Geometry check sheet. Reference: the model listing, model coordinates, mm. Give positions to 0.01 mm unless a question says otherwise; leave off trailing zeros. Loops run counter-clockwise (first coordinate to the right, second up) from the corner with the lowest first, then second, coordinate; pieces in that order, holes last. Notation, with made-up numbers: (-19, 36.25) -> (-9, 36.25) arc R24 cw to (-9, 64.25) -> close; hole circle Ø8 at (11.25, 69.5). An arc over 180 degrees is marked (long way). Answer as a JSON object with one key per item and string values.
from build123d import *

# Parameters (mm, degrees)
BOSS_EXTRUDE1_DEPTH = 1.15
CUT_EXTRUDE1_REACH  = 3.15
SKETCH2_R           = 1.55
SKETCH3_W           = 5.45
SKETCH3_H           = 4.15
BOSS_EXTRUDE2_DEPTH = 2.3
SKETCH4_W           = 9.718661505
SKETCH4_H           = 9.252165754
SKETCH4_W_2         = 4.664957522
SKETCH4_H_2         = 2.876723805
SKETCH4_W_3         = 4.081837833
SKETCH4_H_3         = 2.798974514
SKETCH4_W_4         = 4.159587124
SKETCH4_H_4         = 1.593860487
SKETCH4_W_5         = 2.64347593
SKETCH4_H_5         = 0.971866151
BOSS_EXTRUDE3_DEPTH = 1


with BuildPart() as part:
    # Sketch1 → Boss-Extrude1 (new body)
    with BuildSketch(Plane(origin=(0, 0, 0), x_dir=(1, 0, 0), z_dir=(0, 1, 0))):
        with BuildLine():
            Line((-19.425, 20.3), (19.425, 20.3))
            ThreePointArc((19.425, 20.3), (20.839213562, 19.714213562), (21.425, 18.3))
            Line((21.425, 18.3), (21.425, -18.3))
            ThreePointArc((21.425, -18.3), (20.839213562, -19.714213562), (19.425, -20.3))
            Line((19.425, -20.3), (-19.425, -20.3))
            ThreePointArc((-19.425, -20.3), (-20.839213562, -19.714213562), (-21.425, -18.3))
            Line((-21.425, -18.3), (-21.425, 18.3))
            ThreePointArc((-21.425, 18.3), (-20.839213562, 19.714213562), (-19.425, 20.3))
        make_face()
    extrude(amount=BOSS_EXTRUDE1_DEPTH)

    # Sketch2 → Cut-Extrude1 (cut, up to next)
    with BuildSketch(Plane(origin=(0, 1.15, 0), x_dir=(1, 0, 0), z_dir=(0, 1, 0)), mode=Mode.PRIVATE) as cut_extrude1_sk1:
        with Locations((-13.925, 12.95)):
            Circle(SKETCH2_R)
    cut_extrude1_tool1 = extrude(cut_extrude1_sk1.sketch, amount=-CUT_EXTRUDE1_REACH, mode=Mode.PRIVATE) & part.part
    add(cut_extrude1_tool1.solids().sort_by_distance((-13.925, 1.15, -12.95))[0], mode=Mode.SUBTRACT)
    # Sketch2 → Cut-Extrude1 (cut, up to next)
    with BuildSketch(Plane(origin=(0, 1.15, 0), x_dir=(1, 0, 0), z_dir=(0, 1, 0)), mode=Mode.PRIVATE) as cut_extrude1_sk2:
        with Locations((13.925, -12.95)):
            Circle(SKETCH2_R)
    cut_extrude1_tool2 = extrude(cut_extrude1_sk2.sketch, amount=-CUT_EXTRUDE1_REACH, mode=Mode.PRIVATE) & part.part
    add(cut_extrude1_tool2.solids().sort_by_distance((13.925, 1.15, 12.95))[0], mode=Mode.SUBTRACT)

    # Sketch3 → Boss-Extrude2 (add)
    with BuildSketch(Plane(origin=(0, 1.15, 0), x_dir=(1, 0, 0), z_dir=(0, 1, 0))):
        with Locations((-9.84, -9.405)):
            Rectangle(SKETCH3_W, SKETCH3_H)
    extrude(amount=BOSS_EXTRUDE2_DEPTH)

    # Sketch4 → Boss-Extrude3 (add)
    with BuildSketch(Plane(origin=(0, 1.15, 0), x_dir=(1, 0, 0), z_dir=(0, 1, 0))):
        with Locations((5.908946196, 1.904857655)):
            Rectangle(SKETCH4_W, SKETCH4_H)
        with Locations((6.919686992, 9.329915045)):
            Rectangle(SKETCH4_W_2, SKETCH4_H_2)
        with Locations((-5.656260997, 1.671609779)):
            Rectangle(SKETCH4_W_3, SKETCH4_H_3)
        with Locations((15.025050688, 4.567770907)):
            Rectangle(SKETCH4_W_4, SKETCH4_H_4)
        with Locations((14.99993444, 2.629590434)):
            Rectangle(SKETCH4_W_5, SKETCH4_H_5)
        with Locations((14.99993444, 0.91910601)):
            Rectangle(SKETCH4_W_5, SKETCH4_H_5)
        with Locations((15.025050688, -1.030178119)):
            Rectangle(SKETCH4_W_4, SKETCH4_H_4)
    extrude(amount=BOSS_EXTRUDE3_DEPTH)


solid = part.part
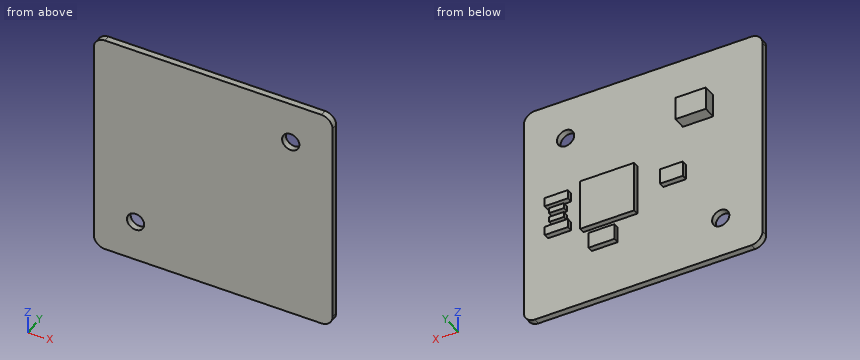
1) Section check B-B on x = 7.5. Record the cut outline in (y, z).
Geometry check:
{"outline": "(0, -20.3) -> (1.15, -20.3) -> (1.15, -10.77) -> (2.15, -10.77) -> (2.15, -7.89) -> (1.15, -7.89) -> (1.15, -6.53) -> (2.15, -6.53) -> (2.15, 2.72) -> (1.15, 2.72) -> (1.15, 20.3) -> (0, 20.3) -> close"}
2) Section check D-D on x = -11. Record the cut outline in (y, z).
Geometry check:
{"outline": "(0, -20.3) -> (1.15, -20.3) -> (1.15, 7.33) -> (3.45, 7.33) -> (3.45, 11.48) -> (1.15, 11.48) -> (1.15, 20.3) -> (0, 20.3) -> close"}
3) Material ranges on line 1 along Z through (x, y) = (6, 2.05); line 2 along X through (y, z) = (0.95, -12.95) (3 decimals); line 3 along X through (y, z) = (0.35, 12.95) (3 decimals), recorded low to high. Write a range as from..to.
Geometry check:
{"line 1": "z = -10.77..-7.89, -6.53..2.72", "line 2": "x = -21.425..-15.475, -12.375..21.425", "line 3": "x = -21.425..12.375, 15.475..21.425"}
4) Depth check by flat-ended pin: P1, Ø0.8, axis at x = 15.5, y = 1.5, coming from the -Z side; P2, Ø0.8, axis at x = 15.5, y = 2, coming from the +Z side; P3, Ø8, axis at x = 6, z = 14.5, coming from the +Y side; P4, Ø0.7, axis at y = 2.5, z = 9.5, coming from the +X side (3 decimals). Enter the tip coordinate at first touch or a pass-through.
Geometry check:
{"P1": "stops at z = -20.3", "P2": "stops at z = 1.83", "P3": "stops at y = 1.15", "P4": "stops at x = -7.115"}
5) Section check A-A on z = 12.95. Record the cut outline in (x, y) (3 decimals), plus the area to 3 significant figures.
Geometry check:
{"outline": "(-21.425, 0) -> (12.375, 0) -> (12.375, 1.15) -> (-21.425, 1.15) -> close; (15.475, 0) -> (21.425, 0) -> (21.425, 1.15) -> (15.475, 1.15) -> close", "area": "45.7 mm2"}
6) Section check C-C on z = -4.5. Record the cut outline in (x, y) (3 decimals).
Geometry check:
{"outline": "(-21.425, 0) -> (21.425, 0) -> (21.425, 1.15) -> (17.105, 1.15) -> (17.105, 2.15) -> (12.945, 2.15) -> (12.945, 1.15) -> (10.768, 1.15) -> (10.768, 2.15) -> (1.05, 2.15) -> (1.05, 1.15) -> (-21.425, 1.15) -> close"}
